from build123d import *

# Parameters (mm, degrees)
F4_DEPTH  = 30.001
F5_W      = 6
F5_H      = 7
F6_DEPTH  = 13
F7_W      = 50.3954237082
F7_H      = 8.0328645855
F8_DEPTH  = 30.001
F9_W      = 10
F9_H      = 4
F10_DEPTH = 2


with BuildPart() as f1:
    # F0 (on Right) → F1 (revolve)
    with BuildSketch(Plane.YZ):
        with BuildLine():
            Line((-30, 0), (0, 0))
            ThreePointArc((0, 0), (-15, 15), (-30, 0))
        make_face()
    revolve(axis=Axis((0, -15, 0), (0, -1, 0)))

    # F3 (on offset) → F4 (cut, through all)
    with BuildSketch(Plane.XY.offset(15)):
        with BuildLine():
            Line((15, 0), (0, 0))
            Line((0, 0), (-15, 0))
            ThreePointArc((-15, 0), (0, -3), (15, 0))
        make_face()
    extrude(amount=-F4_DEPTH, mode=Mode.SUBTRACT)

    # F5 (on Front) → F6 (cut)
    with BuildSketch(Plane.XZ):
        Rectangle(F5_W, F5_H)
    extrude(amount=F6_DEPTH, mode=Mode.SUBTRACT)

    # F7 (on Front) → F8 (cut, through all)
    with BuildSketch(Plane.XZ):
        with Locations((-1.7276192084, 13.5164322928)):
            Rectangle(F7_W, F7_H)
    extrude(amount=F8_DEPTH, mode=Mode.SUBTRACT)

    # F9 (on face) → F10 (join)
    with BuildSketch(Plane.XY.offset(9.5)):
        with Locations((0, -15)):
            Rectangle(F9_W, F9_H)
        Polygon((-5, -17), (-5, -13), (-5, -10), (-10, -15), (-5, -20), align=None)
        Polygon((5, -10), (5, -13), (5, -17), (5, -20), (10, -15), align=None)
    extrude(amount=F10_DEPTH)


solid = f1.part
Could you check a few things on this model? Use its own coordinates, in mm. A direction names the side the tool comes from. Coordinates: 2 decimals unless noted, no trailing zeros. Order: outer loops, then holes, each group sorted by start corner. A loop starts at its lowest first (then second) coordinate and runs counter-clockwise, first axis right, second up. Notation, with made-up numbers: (-38.75, 43) -> (-10.75, 43) arc R23 ccw to (-10.75, 53) -> close; hole circle Ø6 at (4.25, 55.5). An arc over 180 degrees is marked (long way). One line per item, written item: value. Start each with the question number.
1) If I drill on L1, parallel to Y at x = 3.25, z = 10.25; L2, parallel to X at y = -3.5, z = -0.5; L3, parallel to Z at x = 2, y = -4.5, over which ranges is the centre line in solid material (lowest first)? Write a range as [from, to].
2) I'm going to push flat-ended pins straight in: pin 1 (1.6 mm diameter, centred on y = -18, z = 10.5, fed in from -X); pin 2 (5 mm diameter, centred on x = 1, y = -6.5, fed in from +Z); pin 3 (0.6 mm diameter, centred on x = 2.5, z = 11, fed in from -Y). Where does each tip first touch, or does it pass through?
3) We'd pull the mould along X, two halves only. Please class faces 5 (the flat face through (8, -13, 10)), 6 (the flat face through (0, -15, 11.5)), 7 (the flat face through (0, -8, -3.5)): +X half, -X half, draft (parallel to the pull), parting line (faces both ways), or undercut.
4) Which directions (+Z, -Z, +X, -X, +Y, -Y) give clear straight access to the entire face, cutting with the end or side of a thin tool? Please do faces 1 (the flat face through (0, -13, 10)), 2 (the flat face through (3, -8, 0)), 3 (the flat face through (5, -18, 10)), 4 (the flat face through (-7, -12, 10)).
5) Imagine slicing it at D-D on y = -19.25. List the corners of the cut face in (x, z) for me, plus the area to 3 significant figures.
6) Imagine slicing it at A-A on y = -11.75. List the corners of the cut face in (x, z) for me, plus the area to 3 significant figures.
7) Imagine slicing it at C-C on z = 2. List the corners of the cut face in (x, y) for me.
Answer list:
1. L1: y = [-17, -13]
1. L2: x = [-9.62, -3], [3, 9.62]
1. L3: z = [-10.52, -3.5], [3.5, 9.5]
2. pin 1: stops at x = -7.8
2. pin 2: stops at z = 9.5
2. pin 3: stops at y = -17
3. face 5: +X half
3. face 6: draft
3. face 7: undercut
4. face 1: +Z, +Y
4. face 2: +Y
4. face 3: +Z, -Y
4. face 4: +Z, -X, +Y
5. outline: (-10.8, 9.5) arc R14.39 ccw (long way) to (10.8, 9.5) -> (5.75, 9.5) -> (5.75, 11.5) -> (5, 11.5) -> (5, 9.5) -> (-5, 9.5) -> (-5, 11.5) -> (-5.75, 11.5) -> (-5.75, 9.5) -> close
5. area: 580 mm2
6. outline: (-11.14, 9.5) arc R14.64 ccw (long way) to (11.14, 9.5) -> (6.75, 9.5) -> (6.75, 11.5) -> (5, 11.5) -> (5, 9.5) -> (-5, 9.5) -> (-5, 11.5) -> (-6.75, 11.5) -> (-6.75, 9.5) -> close; hole (-3, -3.5) -> (3, -3.5) -> (3, 3.5) -> (-3, 3.5) -> close
6. area: 559 mm2
7. outline: (-7.64, -2.25) arc R14.87 ccw (long way) to (7.64, -2.25) arc R39 cw to (3, -2.88) -> (3, -13) -> (-3, -13) -> (-3, -2.88) arc R39 cw to start
